Geometry: final body of the model. Coordinates: model frame, mm. Give positions to 0.01 mm unless a question says otherwise; leave off trailing zeros. Loops run counter-clockwise (first coordinate to the right, second up) from the corner with the lowest first, then second, coordinate; pieces in that order, holes last.
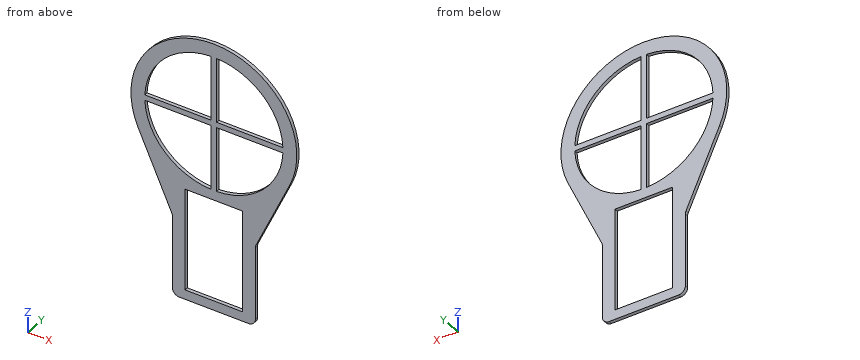
from build123d import *

# Parameters (mm, degrees)
SKETCH1_R           = 76.2
SKETCH1_W           = 76.2
SKETCH1_H           = 76.2
BOSS_EXTRUDE1_DEPTH = 3.175
FILLET1_R           = 6.35
CUT_EXTRUDE1_DEPTH  = 3.175
SKETCH3_W           = 52.989505278
SKETCH3_H           = 96.128397395
CUT_EXTRUDE2_DEPTH  = 3.175


with BuildPart() as part:
    # Sketch1 → Boss-Extrude1 (new body)
    with BuildSketch(Plane(origin=(0, 0, 0), x_dir=(1, 0, 0), z_dir=(0, 1, 0))):
        Circle(SKETCH1_R)
        with BuildLine():
            Line((38.1, 101.6), (-38.1, 101.6))
            Line((-38.1, 101.6), (-69.5842745, 31.055897063))
            ThreePointArc((-69.5842745, 31.055897063), (0, 76.2), (69.5842745, 31.055897063))
            Line((69.5842745, 31.055897063), (38.1, 101.6))
        make_face()
        with Locations((0, 139.7)):
            Rectangle(SKETCH1_W, SKETCH1_H)
    extrude(amount=BOSS_EXTRUDE1_DEPTH)

    # Fillet1
    fillet1_edges = [part.edges().sort_by_distance(p)[0] for p in [
        (-38.1, 1.5875, -101.6),
        (-38.1, 1.5875, -177.8),
        (38.1, 1.5875, -177.8),
        (38.1, 1.5875, -101.6),
    ]]
    fillet(fillet1_edges, radius=FILLET1_R)

    # Sketch2 → Cut-Extrude1 (cut)
    with BuildSketch(Plane(origin=(0, 3.175, 0), x_dir=(1, 0, 0), z_dir=(0, 1, 0))):
        with BuildLine():
            Line((-63.449179664, 2.54), (-2.54, 2.54))
            Line((-2.54, 2.54), (-2.54, 63.449179664))
            ThreePointArc((-2.54, 63.449179664), (-44.901280605, 44.901280605), (-63.449179664, 2.54))
        make_face()
        with BuildLine():
            Line((2.54, 63.449179664), (2.54, 2.54))
            Line((2.54, 2.54), (63.449179664, 2.54))
            ThreePointArc((63.449179664, 2.54), (44.901280605, 44.901280605), (2.54, 63.449179664))
        make_face()
        with BuildLine():
            Line((63.449179664, -2.54), (2.54, -2.54))
            Line((2.54, -2.54), (2.54, -63.449179664))
            ThreePointArc((2.54, -63.449179664), (44.901280605, -44.901280605), (63.449179664, -2.54))
        make_face()
        with BuildLine():
            Line((-2.54, -63.449179664), (-2.54, -2.54))
            Line((-2.54, -2.54), (-63.449179664, -2.54))
            ThreePointArc((-63.449179664, -2.54), (-44.901280605, -44.901280605), (-2.54, -63.449179664))
        make_face()
    extrude(amount=-CUT_EXTRUDE1_DEPTH, mode=Mode.SUBTRACT)

    # Sketch3 → Cut-Extrude2 (cut)
    with BuildSketch(Plane(origin=(0, 3.175, 0), x_dir=(1, 0, 0), z_dir=(0, 1, 0))):
        with Locations((0, 120.773321073)):
            Rectangle(SKETCH3_W, SKETCH3_H)
    extrude(amount=-CUT_EXTRUDE2_DEPTH, mode=Mode.SUBTRACT)


solid = part.part
Item 1: Section query A-A on x = 0. Return loops of the section in (y, z) (3 decimals).
Values follow:
outline: (0, -177.8) - (3.175, -177.8) - (3.175, -168.838) - (0, -168.838) - close; (0, -72.709) - (3.175, -72.709) - (3.175, 76.2) - (0, 76.2) - close
Item 2: Section query D-D on x = 61. Return loops of the section in (y, z) (3 decimals).
Values follow:
outline: (0, -50.29) - (3.175, -50.29) - (3.175, -17.642) - (0, -17.642) - close; (0, -2.54) - (3.175, -2.54) - (3.175, 2.54) - (0, 2.54) - close; (0, 17.642) - (3.175, 17.642) - (3.175, 45.667) - (0, 45.667) - close
Item 3: Pin query (flat end, axial travel): pin 1 (1 mm diameter, centred on y = 1, z = -128, fed in from +X); pin 2 (1 mm diameter, centred on y = 1, z = -25.5, fed in from -X); pin 3 (1.6 mm diameter, centred on y = 2, z = -146, fed in from -X). Return the tip coordinate at first contact, or that it passes through.
Values follow:
pin 1: stops at x = 38.1
pin 2: stops at x = -71.98
pin 3: stops at x = -38.1
Item 4: Ray query, probe 1 along X at (y, z) = (1.2, -115.5); probe 2 along X at (y, z) = (1.2, -23.5); probe 3 along Z at (x, y) = (-22.5, 1.65). Return the intervals inside material, ascending.
Values follow:
probe 1: x = -38.1 to -26.49, 26.49 to 38.1
probe 2: x = -72.49 to -58.99, -2.54 to 2.54, 58.99 to 72.49
probe 3: z = -177.8 to -168.84, -72.71 to -59.38, -2.54 to 2.54, 59.38 to 72.8
Item 5: Section query B-B on z = -48. Return loops of the section in (x, y) (3 decimals), plus the area to 3 significant figures.
Values follow:
outline: (-62.022, 0) - (-41.572, 0) - (-41.572, 3.175) - (-62.022, 3.175) - close; (-2.54, 0) - (2.54, 0) - (2.54, 3.175) - (-2.54, 3.175) - close; (41.572, 0) - (62.022, 0) - (62.022, 3.175) - (41.572, 3.175) - close
area: 146 mm2
Item 6: Section query C-C on y = 2.05. Return loops of the section in (x, z), plus the area to 3 significant figures.
Values follow:
outline: (-69.58, -31.06) - (-38.65, -100.36) arc R6.35 cw to (-38.1, -102.95) - (-38.1, -171.45) arc R6.35 ccw to (-31.75, -177.8) - (31.75, -177.8) arc R6.35 ccw to (38.1, -171.45) - (38.1, -102.95) arc R6.35 cw to (38.65, -100.36) - (69.58, -31.06) arc R76.2 ccw (long way) to start; hole (-63.45, -2.54) arc R63.5 ccw to (-2.54, -63.45) - (-2.54, -2.54) - close; hole (-63.45, 2.54) - (-2.54, 2.54) - (-2.54, 63.45) arc R63.5 ccw to start; hole (-26.49, -168.84) - (26.49, -168.84) - (26.49, -72.71) - (-26.49, -72.71) - close; hole (2.54, -63.45) arc R63.5 ccw to (63.45, -2.54) - (2.54, -2.54) - close; hole (2.54, 2.54) - (63.45, 2.54) arc R63.5 ccw to (2.54, 63.45) - close
area: 10,600 mm2
